from build123d import *

# Parameters (mm, degrees)
SKETCH_1_R          = 1.9
SKETCH_1_R_2        = 1.5
SKETCH_1_R_3        = 2
EXTRUDE_1_DEPTH     = 4
SKETCH_2_R          = 2
CUT_EXTRUDE_1_DEPTH = 171.226319939


with BuildPart() as part:
    # 草图1 → 凸台-拉伸1 (new body)
    with BuildSketch(Plane.XY):
        with BuildLine():
            Line((168.953879648, -0.909966618), (168.931448962, -1.108701692))
            ThreePointArc((168.931448962, -1.108701692), (165.63568786, -7.017052255), (159.155370177, -8.960279039))
            ThreePointArc((159.155370177, -8.960279039), (85.523468127, -4.894349995), (11.798026408, -6.552065898))
            ThreePointArc((11.798026408, -6.552065898), (8.320365096, -7.182704729), (5.086801975, -8.609555486))
            ThreePointArc((5.086801975, -8.609555486), (0.664725554, -9.977882538), (-3.899782135, -9.208240836))
            ThreePointArc((-3.899782135, -9.208240836), (-27.893230932, -3.454367969), (-52.455418381, -5.797781267))
            ThreePointArc((-52.455418381, -5.797781267), (-59.85652595, -1.304263697), (-55.061728395, 5.905313947))
            ThreePointArc((-55.061728395, 5.905313947), (-30.640902591, 11.356196493), (-6.759259259, 18.823188207))
            ThreePointArc((-6.759259259, 18.823188207), (-3.365966263, 19.714722192), (0.130908203, 19.999571571))
            ThreePointArc((0.130908203, 19.999571571), (80.824453525, 16.963385457), (161.173821166, 8.923124109))
            ThreePointArc((161.173821166, 8.923124109), (167.057974161, 5.584353207), (168.953879648, -0.909966618))
        make_face()
        with Locations((32, 7)):
            Circle(SKETCH_1_R, mode=Mode.SUBTRACT)
        with Locations((135, 2.8)):
            Circle(SKETCH_1_R, mode=Mode.SUBTRACT)
        with Locations((-54, 0)):
            Circle(SKETCH_1_R_2, mode=Mode.SUBTRACT)
        Circle(SKETCH_1_R_3, mode=Mode.SUBTRACT)
        with Locations((160, 0)):
            Circle(SKETCH_1_R_2, mode=Mode.SUBTRACT)
    extrude(amount=EXTRUDE_1_DEPTH)

    # 草图2 → 切除-拉伸1 (cut, through all)
    with BuildSketch(Plane.XY.offset(4)):
        with Locations((160, 0)):
            Circle(SKETCH_2_R)
    extrude(amount=-CUT_EXTRUDE_1_DEPTH, mode=Mode.SUBTRACT)


solid = part.part
Can you work these out from the model? Positions are in its coordinate system, mm. A direction names the side the tool comes from. Give positions to 0.01 mm unless a question says otherwise; leave off trailing zeros. Loops run counter-clockwise (first coordinate to the right, second up) from the corner with the lowest first, then second, coordinate; pieces in that order, holes last. Notation, with made-up numbers: (42, 80) - (64, 80) arc R30 ccw to (64, 111) - close; hole circle Ø3 at (-28.75, 0.5). An arc over 180 degrees is marked (long way). One line per item, written item: value.
(1) On a 3-axis mill with a long thin cutter (end or side, diameter ignored), from which of +Z, -Z, +X, -X, +Y, -Y can I reach the whole of each face in a straight line? I mean faces 1 (the face through (79.7, 17.04, 1.97)), 2 (the face through (8.368, -7.168, 1.972)). Say none if no direction works.
Verdict:
face 1: +Z, -Z, +X, +Y
face 2: +Z, -Z, -Y
(2) I'm going to push flat-ended pins straight in: pin 1 (5 mm diameter, centred on x = 160, y = 0, fed in from -Z); pin 2 (3 mm diameter, centred on x = 32, y = 7, fed in from -Z); pin 3 (1 mm diameter, centred on y = 6.5, z = 2.5, fed in from +X); pin 4 (1 mm diameter, centred on y = -2, z = 0.5, fed in from +X). Where does each tip first touch, or does it pass through?
Verdict:
pin 1: z = 0
pin 2: through
pin 3: x = 166.71
pin 4: x = 168.87
(3) If we section it at D-D, the plane x = 32: List the corners of the cut face in (y, z) for me, plus the area to 3 significant figures.
Verdict:
outline: (-5.53, 0) - (5.1, 0) - (5.1, 4) - (-5.53, 4) - close; (8.9, 0) - (19.4, 0) - (19.4, 4) - (8.9, 4) - close
area: 84.5 mm^2
(4) If we section it at B-B, the plane z = 0.6: List the corners of the cut face in (x, y) for me.
Verdict:
outline: (-55.06, 5.91) arc R6 ccw (long way) to (-52.46, -5.8) arc R75 cw to (-3.9, -9.21) arc R10 ccw to (5.09, -8.61) arc R15 cw to (11.8, -6.55) arc R950 cw to (159.16, -8.96) arc R9 ccw to (168.93, -1.11) - (168.95, -0.91) arc R9 ccw to (161.17, 8.92) arc R1300 ccw to (0.13, 20) arc R20 ccw to (-6.76, 18.82) arc R300 cw to start; hole circle Ø3 at (-54, 0); hole circle Ø4 at (0, 0); hole circle Ø3.8 at (32, 7); hole circle Ø3.8 at (135, 2.8); hole circle Ø4 at (160, 0)
(5) If we section it at A-A, the plane x = 135: List the corners of the cut face in (y, z) for me, plus the area to 3 significant figures.
Verdict:
outline: (-6.99, 0) - (0.9, 0) - (0.9, 4) - (-6.99, 4) - close; (4.7, 0) - (12.1, 0) - (12.1, 4) - (4.7, 4) - close
area: 61.2 mm^2
(6) I need wall thicknesses on line 1 along Y through (x, z) = (0, 1.25); line 2 along X through (y, z) = (3.75, 3.75); line 3 along Y through (x, z) = (-54, 1.4). Which ranges of each line are inside material? Lowest first, please.
Verdict:
line 1: -10 to -2, 2 to 20
line 2: -58.68 to 133.35, 136.65 to 168.18
line 3: -6 to -1.5, 1.5 to 6.1
